Work out the finished part from the listing and answer in its coordinate system (mm). Face numbers are marked on the shaded views. A direction names the side the tool comes from. Coordinates: 2 decimals unless noted, no trailing zeros. Order: outer loops, then holes, each group sorted by start corner. A loop starts at its lowest first (then second) coordinate and runs counter-clockwise, first axis right, second up.
1. A tool of negligible diameter and unlimited length cuts with its end or side. For the marked faces 5 and 6, from which of +Z, -Z, +X, -X, +Y, -Y can it reach the whole face along a straight path? Write none if from no direction.
2. Find the intervals of material crossed by probe 1 along X at (y, z) = (0, -5); probe 2 along X at (y, z) = (2.5, 3); probe 3 along Y at (x, z) = (-2, -16), in increasing order.
3. Flat-ended cylindrical pins translate along their axes: pin 1 Ø8.5 at (x, y) = (0, 0) entering from -Z; pin 2 Ø2.5 at (y, z) = (7.5, 3) entering from -X; pin 3 Ø2.5 at (y, z) = (-6.5, 4.5) entering from +X; pin 4 Ø5 at (x, z) = (0, -20) entering from +Y. Find the tip coordinate at first contact, or state that the pin passes through.
4. Determine the mould class of the marked faces 1, 2, 3 and 4 for opening direction X: +X half, -X half, draft (parallel to the pull), parting line (faces both ways), or undercut.
5. The part is cut by section B-B, the plane z = -20. Give the vertices of the cut face in (x, y), then the cut area to 3 significant figures.
6. The part is cut by section A-A, the plane z = -2.5. Give the vertices of the cut face in (x, y).
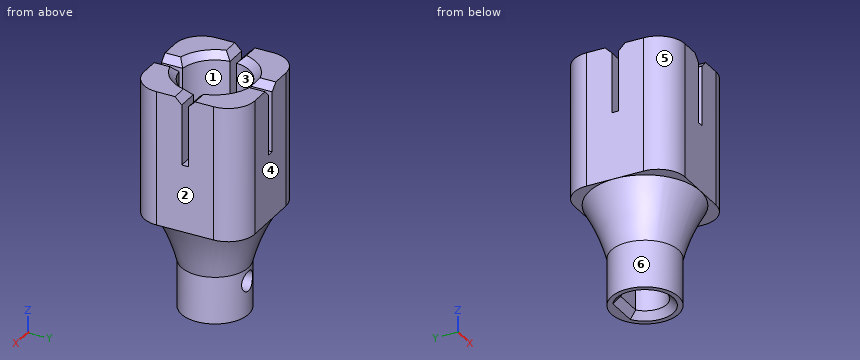
```python
from build123d import *

# Parameters (mm, degrees)
BOSS_EXTRUDE1_DEPTH = 10
SKETCH12_R          = 5
BOSS_EXTRUDE3_DEPTH = 15
CUT_EXTRUDE3_DEPTH  = 40
SKETCH14_R          = 1.5
CUT_EXTRUDE4_DEPTH  = 12
CHAMFER5_SIZE       = 1
SKETCH10_W          = 1
SKETCH10_H          = 10
SKETCH10_W_2        = 10
SKETCH10_H_2        = 1
CUT_EXTRUDE5_DEPTH  = 25
SKETCH16_R          = 5.1
CUT_EXTRUDE6_DEPTH  = 25
CHAMFER6_SIZE       = 1
CHAMFER7_SIZE       = 1


with BuildPart() as part:
    # Sketch2 → Boss-Extrude1 (new body, symmetric)
    with BuildSketch(Plane.XY):
        with BuildLine():
            Line((4.25, -8.25), (-4.25, -8.25))
            ThreePointArc((-4.25, -8.25), (-7.078427125, -7.078427125), (-8.25, -4.25))
            Line((-8.25, -4.25), (-8.25, 4.25))
            ThreePointArc((-8.25, 4.25), (-7.078427125, 7.078427125), (-4.25, 8.25))
            Line((-4.25, 8.25), (4.25, 8.25))
            ThreePointArc((4.25, 8.25), (7.078427125, 7.078427125), (8.25, 4.25))
            Line((8.25, 4.25), (8.25, -4.25))
            ThreePointArc((8.25, -4.25), (7.078427125, -7.078427125), (4.25, -8.25))
        make_face()
    extrude(amount=BOSS_EXTRUDE1_DEPTH, both=True)

    # Sketch12 → Boss-Extrude3 (add)
    with BuildSketch(Plane(origin=(0, 0, -10), x_dir=(-1, 0, 0), z_dir=(0, 0, -1))):
        Circle(SKETCH12_R)
    extrude(amount=BOSS_EXTRUDE3_DEPTH)

    # Sketch13 → Cut-Extrude3 (cut)
    with BuildSketch(Plane(origin=(0, 0, -25), x_dir=(-1, 0, 0), z_dir=(0, 0, -1))):
        with BuildLine():
            Line((-2.076655966, 2.5), (2.076655966, 2.5))
            ThreePointArc((2.076655966, 2.5), (0, -3.25), (-2.076655966, 2.5))
        make_face()
    extrude(amount=-CUT_EXTRUDE3_DEPTH, mode=Mode.SUBTRACT)

    # Sketch14 → Cut-Extrude4 (cut)
    with BuildSketch(Plane(origin=(0, 0, 0), x_dir=(1, 0, 0), z_dir=(0, 1, 0))):
        with Locations((0, 20)):
            Circle(SKETCH14_R)
    extrude(amount=CUT_EXTRUDE4_DEPTH, mode=Mode.SUBTRACT)

    # Chamfer5
    chamfer5_edges = [part.edges().sort_by_distance(p)[0] for p in [
        (0, 2.5, -25),
        (0, -3.25, -25),
    ]]
    chamfer(chamfer5_edges, length=CHAMFER5_SIZE)

    # Sketch10 → Cut-Extrude5 (cut)
    with BuildSketch(Plane.XY):
        with Locations((0, 8)):
            Rectangle(SKETCH10_W, SKETCH10_H)
        with Locations((8, 0)):
            Rectangle(SKETCH10_W_2, SKETCH10_H_2)
        with Locations((0, -8)):
            Rectangle(SKETCH10_W, SKETCH10_H)
        with Locations((-8, 0)):
            Rectangle(SKETCH10_W_2, SKETCH10_H_2)
    extrude(amount=CUT_EXTRUDE5_DEPTH, mode=Mode.SUBTRACT)

    # Sketch16 → Cut-Extrude6 (cut)
    with BuildSketch(Plane.XY):
        Circle(SKETCH16_R)
    extrude(amount=CUT_EXTRUDE6_DEPTH, mode=Mode.SUBTRACT)

    # Sketch56 → Revolve3 (revolve)
    with BuildSketch(Plane(origin=(0, 0, 0), x_dir=(0, 0, -1), z_dir=(1, 0, 0))):
        with BuildLine():
            Line((10, 5), (10, 8.25))
            ThreePointArc((10, 8.25), (13.882456458, 6.335662049), (18, 5))
            Line((18, 5), (10, 5))
        make_face()
    revolve(axis=Axis((0, 0, 0), (0, 0, -1)))

    # Chamfer6
    chamfer6_edges = [part.edges().sort_by_distance(p)[0] for p in [
        (-3.606244584, -3.606244584, 10),
        (3.606244584, -3.606244584, 10),
        (3.606244584, 3.606244584, 10),
        (-3.606244584, 3.606244584, 10),
    ]]
    chamfer(chamfer6_edges, length=CHAMFER6_SIZE)

    # Chamfer7
    chamfer7_edges = [part.edges().sort_by_distance(p)[0] for p in [
        (0.5, 7.164736831, 10),
        (-0.5, 7.164736831, 10),
        (-7.164736831, 0.5, 10),
        (-7.164736831, -0.5, 10),
        (-0.5, -7.164736831, 10),
        (0.5, -7.164736831, 10),
        (7.164736831, -0.5, 10),
        (7.164736831, 0.5, 10),
    ]]
    chamfer(chamfer7_edges, length=CHAMFER7_SIZE)


solid = part.part
```
Geometry says:
1. face 5: +Z, -Z, -X, -Y
1. face 6: -Z
2. probe 1: x = -8.25 to -3.25, 3.25 to 8.25
2. probe 2: x = -8.25 to -4.45, 4.45 to 8.25
2. probe 3: y = -5.2 to -2.56, 2.5 to 5.2
3. pin 1: stops at z = -25
3. pin 2: stops at x = -7.71
3. pin 3: stops at x = 8.12
3. pin 4: stops at y = 5.13
4. face 1: undercut
4. face 2: +X half
4. face 3: undercut
4. face 4: draft
5. outline: (-2.08, 2.5) - (-1.5, 2.5) - (-1.5, 4.77) arc R5 ccw (long way) to (1.5, 4.77) - (1.5, 2.5) - (2.08, 2.5) arc R3.25 cw (long way) to start
5. area: 40.2 mm2
6. outline: (-8.25, -4.25) arc R4 ccw to (-4.25, -8.25) - (4.25, -8.25) arc R4 ccw to (8.25, -4.25) - (8.25, 4.25) arc R4 ccw to (4.25, 8.25) - (-4.25, 8.25) arc R4 ccw to (-8.25, 4.25) - close; hole (-2.08, 2.5) arc R3.25 ccw (long way) to (2.08, 2.5) - close
